from build123d import *

# Parameters (mm, degrees)
SKETCH1_R               = 3.175
SKETCH1_R_2             = 11
BOSS_EXTRUDE1_DEPTH     = 6.35
FILLET3_R               = 2
CUT_EXTRUDE1_REACH      = 111.565
CUT_EXTRUDE1_END_RADIUS = 11
SKETCH2_R               = 1.1303


with BuildPart() as part:
    # Sketch1 → Boss-Extrude1 (new body)
    with BuildSketch(Plane.XY):
        with BuildLine():
            Line((-38.1, -12.7), (-38.1, 12.7))
            Line((-38.1, 12.7), (19.799208724, 12.7))
            Line((19.799208724, 12.7), (49.063216326, -5.044542368))
            ThreePointArc((49.063216326, -5.044542368), (63.185378941, -10.82071629), (66.044603929, -25.808194216))
            Line((66.044603929, -25.808194216), (62.155933896, -32.221324916))
            ThreePointArc((62.155933896, -32.221324916), (47.544550454, -36.615313538), (35.893587146, -26.763678338))
            Line((35.893587146, -26.763678338), (12.7, -12.7))
            Line((12.7, -12.7), (-38.1, -12.7))
        make_face()
        with Locations((-25.4, 0)):
            Circle(SKETCH1_R, mode=Mode.SUBTRACT)
        Circle(SKETCH1_R, mode=Mode.SUBTRACT)
        with Locations((50.8, -20.95)):
            Circle(SKETCH1_R_2, mode=Mode.SUBTRACT)
    extrude(amount=BOSS_EXTRUDE1_DEPTH)

    # Fillet3
    fillet3_edges = [part.edges().sort_by_distance(p)[0] for p in [
        (-38.1, -12.7, 3.175),
        (-38.1, 12.7, 3.175),
        (19.799208724, 12.7, 3.175),
        (12.7, -12.7, 3.175),
    ]]
    fillet(fillet3_edges, radius=FILLET3_R)

    # Cut-Extrude1: up to this cylinder (the profile starts outside it)
    cut_extrude1_end = Plane(origin=(50.8, -20.95, 3.175), z_dir=(0, 0, -1)) * Cylinder(CUT_EXTRUDE1_END_RADIUS, 246.13, mode=Mode.PRIVATE)
    # Sketch2 → Cut-Extrude1 (cut, up to the surface)
    with BuildSketch(Plane(origin=(59.73186838, -36.21905392, 0), x_dir=(0, 0, -1), z_dir=(0.855084093292463, -0.5184893377864259, 0)), mode=Mode.PRIVATE) as cut_extrude1_sk1:
        with Locations(Location((-3.175, 8.425246605, 0), (0, 0, 90))):
            Circle(SKETCH2_R)
    cut_extrude1_tool1 = extrude(cut_extrude1_sk1.sketch, amount=-CUT_EXTRUDE1_REACH, mode=Mode.PRIVATE) - cut_extrude1_end
    add(cut_extrude1_tool1.solids().sort_by_distance((64.100269, -29.01476, 3.175))[0], mode=Mode.SUBTRACT)


solid = part.part
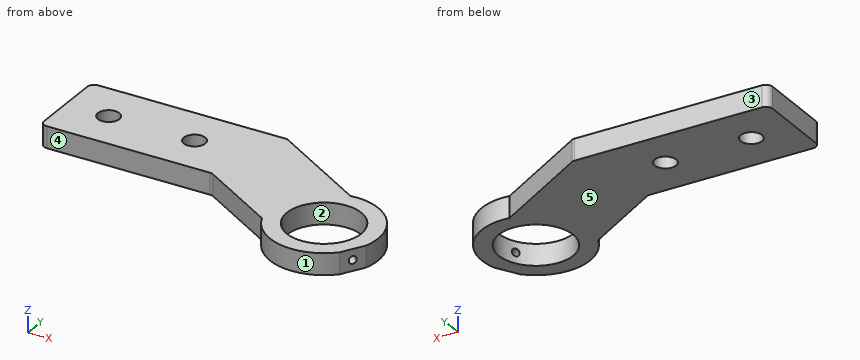
Geometry: final body of the model. Coordinates: model frame, mm. Face numbers are marked on the shaded views. A direction names the side the tool comes from. Coordinates: 2 decimals unless noted, no trailing zeros. Order: outer loops, then holes, each group sorted by start corner. A loop starts at its lowest first (then second) coordinate and runs counter-clockwise, first axis right, second up.
1) Section C-C (y = 0). Return loops of the section in (x, z) (3 decimals), then the cut area to 3 significant figures.
Result sheet:
outline: (-38.1, 0) - (-28.575, 0) - (-28.575, 6.35) - (-38.1, 6.35) - close; (-22.225, 0) - (-3.175, 0) - (-3.175, 6.35) - (-22.225, 6.35) - close; (3.175, 0) - (40.744, 0) - (40.744, 6.35) - (3.175, 6.35) - close
area: 420 mm2
2) Ray query, probe 1 along Y at (x, z) = (50.8, 4.5); probe 2 along Y at (x, z) = (0, 5) (3 decimals); probe 3 along Y at (x, z) = (-22, 1). Return the intervals inside material, ascending.
Result sheet:
probe 1: y = -36.95 to -31.95, -9.95 to -4.95
probe 2: y = -12.7 to -3.175, 3.175 to 12.7
probe 3: y = -12.7 to 12.7
3) Section D-D (x = 31). Return loops of the section in (y, z), then the cut area to 3 significant figures.
Result sheet:
outline: (-23.8, 0) - (5.91, 0) - (5.91, 6.35) - (-23.8, 6.35) - close
area: 189 mm2
4) Draft query along X for the marked faces 1, 2 and 3. Return one class per face: released by +X, released by -X, zero draft, split by the parting line, or undercut.
Result sheet:
face 1: split by the parting line
face 2: undercut
face 3: zero draft
5) Set-up query: the marked faces 4 and 5. Return all of +Z, -Z, +X, -X, +Y, -Y with unobstructed straight access to the full face (end or side cutting, diameter ignored); none if empty.
Result sheet:
face 4: +Z, -Z, -X, -Y
face 5: -Z, +X, -X, +Y, -Y
6) Section B-B (y = -20). Return loops of the section in (x, z), then the cut area to 3 significant figures.
Result sheet:
outline: (24.74, 0) - (39.84, 0) - (39.84, 6.35) - (24.74, 6.35) - close; (61.76, 0) - (66.77, 0) - (66.77, 6.35) - (61.76, 6.35) - close
area: 128 mm2
7) First-contact query: P1, Ø1, axis at x = -17.5, z = 3, coming from the -Y side; P2, Ø1.5, axis at x = 54, z = 2.5, coming from the +Y side. Flat tips, straight axial feed; report the tip coordinate or a pass-through.
Result sheet:
P1: stops at y = -12.7
P2: stops at y = -5.14
8) Section A-A (x = 0). Return loops of the section in (y, z) (3 decimals), then the cut area to 3 significant figures.
Result sheet:
outline: (-12.7, 0) - (-3.175, 0) - (-3.175, 6.35) - (-12.7, 6.35) - close; (3.175, 0) - (12.7, 0) - (12.7, 6.35) - (3.175, 6.35) - close
area: 121 mm2
